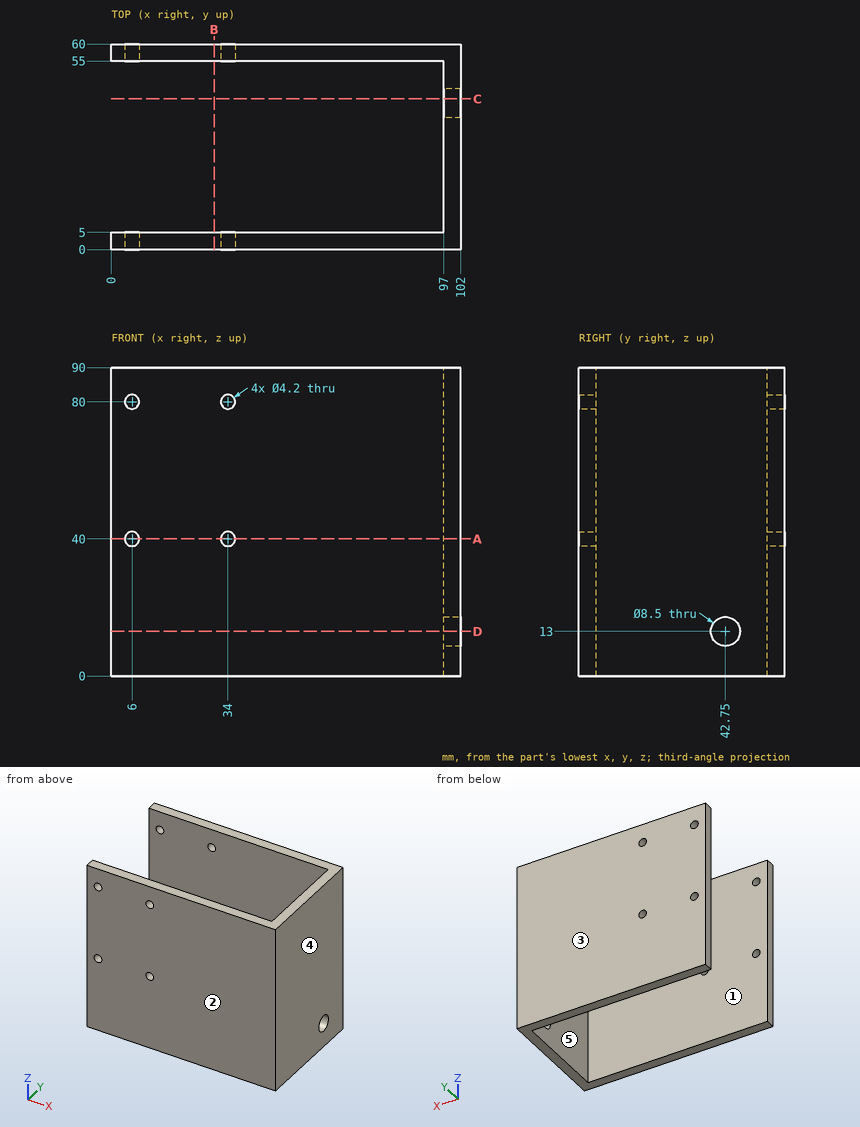
Verification items for this drawing (mm, ordinates from the low corner). A direction names the side the tool comes from. Give positions to 0.01 mm unless a question says otherwise; leave off trailing zeros. Write each loop counter-clockwise with the first axis right and the second up, starting at its lowest first coordinate (ties: lowest second). Pieces come first, ordered by that corner, then holes.
1) Section check C-C, the plane y = 44. Record the boundary of the cut face in (x, z), and give its area (3 significant figures).
2) Section check D-D, the plane z = 13. Record the boundary of the cut face in (x, y).
3) Section check A-A, the plane z = 40. Record the boundary of the cut face in (x, y).
4) Release check for a two-part mould opening along Y. For the marked faces 1, 2 and 3 record: pulls with the +Y half, pulls with the -Y half, needs draft (parallel to the pull), parting line crosses it, or undercut.
5) Gauge pin test, flat ends, axial feed: pin 1 (4 mm diameter, centred on x = 34, z = 40, fed in from -Y); pin 2 (10 mm diameter, centred on y = 32, z = 77, fed in from -X). Record the tip position at first contact, or that the pin passes through.
6) Access from +Z, -Z, +X, -X, +Y, -Y to the whole of each face (thin tool, end or side, straight path). Record for the marked faces 4 and 5.
7) Section check B-B, the plane x = 30. Record the boundary of the cut face in (y, z).
8) Material ranges on L1, parallel to Z at x = 34, y = 3.9; L2, parallel to X at y = 2.8, z = 80; L3, parallel to Y at x = 61.5, z = 66, recorded low to high.
Computed:
1. outline: (97, 0) - (102, 0) - (102, 8.94) - (97, 8.94) - close; (97, 17.06) - (102, 17.06) - (102, 90) - (97, 90) - close
1. area: 409 mm2
2. outline: (0, 0) - (102, 0) - (102, 38.5) - (97, 38.5) - (97, 5) - (0, 5) - close; (0, 55) - (97, 55) - (97, 47) - (102, 47) - (102, 60) - (0, 60) - close
3. outline: (0, 0) - (3.9, 0) - (3.9, 5) - (0, 5) - close; (0, 55) - (3.9, 55) - (3.9, 60) - (0, 60) - close; (8.1, 0) - (31.9, 0) - (31.9, 5) - (8.1, 5) - close; (8.1, 55) - (31.9, 55) - (31.9, 60) - (8.1, 60) - close; (36.1, 0) - (102, 0) - (102, 60) - (36.1, 60) - (36.1, 55) - (97, 55) - (97, 5) - (36.1, 5) - close
4. face 1: undercut
4. face 2: pulls with the -Y half
4. face 3: pulls with the +Y half
5. pin 1: passes through
5. pin 2: stops at x = 97
6. face 4: +Z, -Z, +X, +Y, -Y
6. face 5: +Z, -Z, -X
7. outline: (0, 0) - (5, 0) - (5, 90) - (0, 90) - close; (55, 0) - (60, 0) - (60, 90) - (55, 90) - close
8. L1: z = 0 to 37.9, 42.1 to 77.9, 82.1 to 90
8. L2: x = 0 to 3.9, 8.1 to 31.9, 36.1 to 102
8. L3: y = 0 to 5, 55 to 60
